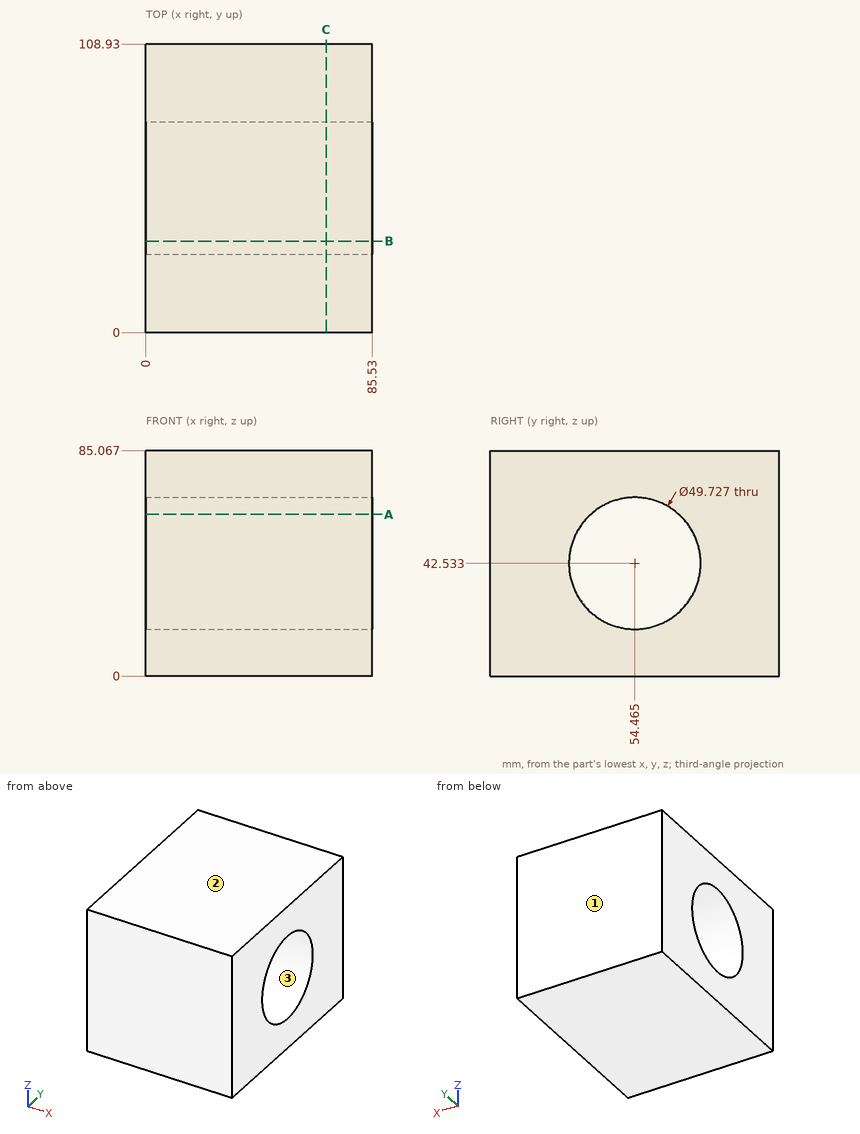
Could you check a few things on this drawing? It's one solid part, dimensions in mm from its lowest x, y, z. Give positions to 0.01 mm unless a question says otherwise; leave off trailing zeros. Loops run counter-clockwise (first coordinate to the right, second up) from the corner with the lowest first, then second, coordinate; pieces in that order, holes last. Notation, with made-up numbers: (44, 56) -> (88, 56) arc R23 cw to (88, 92) -> close; hole circle Ø9 at (71, -30). An arc over 180 degrees is marked (long way). Answer as CSV lines item,"result". Start each with the question number.
(1) If we section it at C-C on x = 68: Write out the boundary of the cut face in (y, z) (1 decimal).
(2) I need wall thicknesses on probe 1 along Z at (x, y) = (12, 32.5) (1 decimal); probe 2 along Y at (x, z) = (22, 56) (1 decimal); probe 3 along Z at (x, y) = (67, 46) (1 decimal). Which ranges of each line are inside material? Lowest first, please.
(3) We'd pull the mould along Y, two halves only. Please class the marked faces 1, 2 and 3: released by +Y, released by -Y, zero draft, split by the parting line, or undercut.
(4) If we section it at B-B on y = 34.5: Write out the boundary of the cut face in (x, z) (1 decimal).
(5) If we section it at A-A on z = 61: Write out the boundary of the cut face in (x, y) (1 decimal).
(6) I'm going to push a flat-ended pin straight in: pin 1 Ø6 at (x, z) = (25.5, 73) entering from -Y. Where does the tip first touch, or does it pass through?
Computed:
1,outline,"(0, 0) -> (108.9, 0) -> (108.9, 85.1) -> (0, 85.1) -> close; hole circle Ø49.7 at (54.5, 42.5)"
2,probe 1,"z = 0 to 30.9, 54.2 to 85.1"
2,probe 2,"y = 0 to 33.6, 75.4 to 108.9"
2,probe 3,"z = 0 to 19.2, 65.9 to 85.1"
3,face 1,"released by +Y"
3,face 2,"zero draft"
3,face 3,"undercut"
4,outline,"(0, 0) -> (85.5, 0) -> (85.5, 27.7) -> (0, 27.7) -> close; (0, 57.4) -> (85.5, 57.4) -> (85.5, 85.1) -> (0, 85.1) -> close"
5,outline,"(0, 0) -> (85.5, 0) -> (85.5, 37.8) -> (0, 37.8) -> close; (0, 71.1) -> (85.5, 71.1) -> (85.5, 108.9) -> (0, 108.9) -> close"
6,pin 1,"stops at y = 0"
